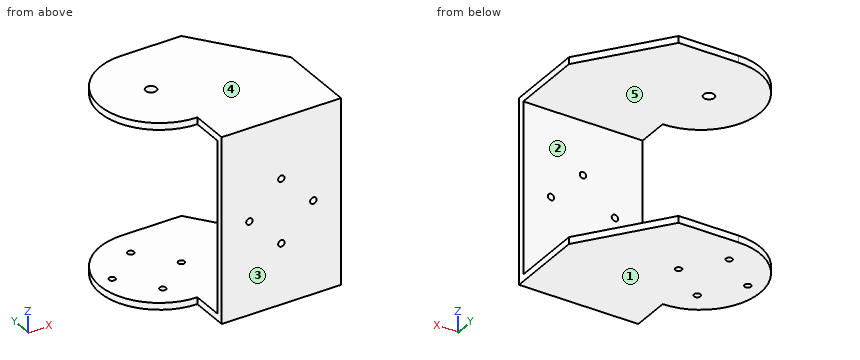
```python
from build123d import *

# Parameters (mm, degrees)
SKETCH1_W           = 28
SKETCH1_H           = 43.264
SKETCH1_R           = 0.75
BOSS_EXTRUDE1_DEPTH = 1.59
SKETCH2_W           = 28
SKETCH2_H           = 1.59
BOSS_EXTRUDE2_DEPTH = 35.41
BOSS_EXTRUDE5_DEPTH = 1.59
BOSS_EXTRUDE6_START = -1.59
BOSS_EXTRUDE6_DEPTH = 1.59
SKETCH9_R           = 0.75
CUT_EXTRUDE3_DEPTH  = 10
SKETCH10_R          = 1.25
CUT_EXTRUDE4_DEPTH  = 10
CUT_EXTRUDE5_REACH  = 65.441


with BuildPart() as part:
    # Sketch1 → Boss-Extrude1 (new body)
    with BuildSketch(Plane(origin=(0, 0, 0), x_dir=(1, 0, 0), z_dir=(0, 1, 0))):
        Rectangle(SKETCH1_W, SKETCH1_H)
        with Locations(Location((0, 7.5, 0), (0, 0, 90))):
            Circle(SKETCH1_R, mode=Mode.SUBTRACT)
        with Locations(Location((0, -7.5, 0), (0, 0, 90))):
            Circle(SKETCH1_R, mode=Mode.SUBTRACT)
        with Locations(Location((7.5, 0, 0), (0, 0, 90))):
            Circle(SKETCH1_R, mode=Mode.SUBTRACT)
        with Locations(Location((-7.5, 0, 0), (0, 0, 90))):
            Circle(SKETCH1_R, mode=Mode.SUBTRACT)
    extrude(amount=BOSS_EXTRUDE1_DEPTH)

    # Sketch2 → Boss-Extrude2 (add)
    with BuildSketch(Plane(origin=(0, 1.59, 0), x_dir=(1, 0, 0), z_dir=(0, 1, 0))):
        with Locations((0, 20.837)):
            Rectangle(SKETCH2_W, SKETCH2_H)
        with Locations((0, -20.837)):
            Rectangle(SKETCH2_W, SKETCH2_H)
    extrude(amount=BOSS_EXTRUDE2_DEPTH)

    # Sketch7 → Boss-Extrude5 (add)
    with BuildSketch(Plane(origin=(0, 0, -21.632), x_dir=(-1, 0, 0), z_dir=(0, 0, -1))):
        with BuildLine():
            Line((14, 37), (14, 9))
            ThreePointArc((14, 9), (28, 23), (14, 37))
        make_face()
    extrude(amount=-BOSS_EXTRUDE5_DEPTH)

    # Sketch8 → Boss-Extrude6 (add)
    with BuildSketch(Plane.XY.offset(21.632).offset(BOSS_EXTRUDE6_START)):
        with BuildLine():
            Line((-14, 37), (-14, 9))
            ThreePointArc((-14, 9), (-28, 23), (-14, 37))
        make_face()
    extrude(amount=BOSS_EXTRUDE6_DEPTH)

    # Sketch9 → Cut-Extrude3 (cut)
    with BuildSketch(Plane(origin=(0, 0, -21.632), x_dir=(-1, 0, 0), z_dir=(0, 0, -1))):
        with Locations((16, 30.5)):
            Circle(SKETCH9_R)
        with Locations((24.5, 24)):
            Circle(SKETCH9_R)
        with Locations((18, 15.5)):
            Circle(SKETCH9_R)
        with Locations((9.5, 22)):
            Circle(SKETCH9_R)
    extrude(amount=-CUT_EXTRUDE3_DEPTH, mode=Mode.SUBTRACT)

    # Sketch10 → Cut-Extrude4 (cut)
    with BuildSketch(Plane.XY.offset(21.632)):
        with Locations((-16, 23)):
            Circle(SKETCH10_R)
    extrude(amount=-CUT_EXTRUDE4_DEPTH, mode=Mode.SUBTRACT)

    # Cut-Extrude5: up to this face of the body (flat: up to its plane)
    cut_extrude5_end = Plane(part.part.faces().sort_by_distance((-4.502841696, 19.512586882, -21.632))[0])
    # Sketch11 → Cut-Extrude5 (cut, up to the picked face)
    with BuildSketch(Plane.XY.offset(21.632), mode=Mode.PRIVATE) as cut_extrude5_sk1:
        Polygon((0, 37), (14, 18.5), (14, 37), align=None)
    cut_extrude5_tool1 = split(extrude(cut_extrude5_sk1.sketch, amount=-CUT_EXTRUDE5_REACH, mode=Mode.PRIVATE), bisect_by=cut_extrude5_end, keep=Keep.BOTH, mode=Mode.PRIVATE)
    add(cut_extrude5_tool1.solids().sort_by(Axis((9.333333, 30.833333, 21.632), (0, 0, -1)))[0], mode=Mode.SUBTRACT)


solid = part.part
```
Work out the finished part from the listing and answer in its coordinate system (mm). Face numbers are marked on the shaded views. A direction names the side the tool comes from. Round coordinates to 2 decimals unless told otherwise and drop trailing zeros. Write each loop counter-clockwise with the first axis right and the second up, starting at its lowest first coordinate (ties: lowest second). Pieces come first, ordered by that corner, then holes.
1) Consider probe 1 along X at (y, z) = (1, 0); probe 2 along Z at (x, y) = (-15, 27); probe 3 along Y at (x, z) = (-13, 18). Determine where each line is inside the solid, lowest interval first.
2) Determine the mould class of the marked faces 3, 4 and 5 for opening direction Z: pulls with the +Z half, pulls with the -Z half, needs draft (parallel to the pull), parting line crosses it, or undercut.
3) A cutting plane is placed at D-D on x = -18. Determine the outline of the cut face in (y, z).
4) A cutting plane is placed at B-B on x = -7.5. Determine the outline of the cut face in (y, z), and give its area (3 significant figures).
5) Which of the six approach directions +Z, -Z, +X, -X, +Y, -Y give full straight-line access (tool end or side, diameter ignored) to the marked faces 1 and 2?
6) Flat-ended cylindrical pins translate along their axes: P1, Ø2.5, axis at y = 4.5, z = -5, coming from the -X side (3 decimals); P2, Ø2, axis at x = -11.5, z = -1.5, coming from the +Y side. Find the tip coordinate at first contact, or state that the pin passes through.
7) A cutting plane is placed at C-C on y = 32. Determine the outline of the cut face in (x, z).
8) A cutting plane is placed at A-A on z = 7.5. Determine the outline of the cut face in (x, y).
Entries:
1. probe 1: x = -14 to -8.25, -6.75 to 6.75, 8.25 to 14
1. probe 2: z = -21.63 to -20.04, 20.04 to 21.63
1. probe 3: y = 0 to 1.59
2. face 3: needs draft
2. face 4: pulls with the +Z half
2. face 5: undercut
3. outline: (9.58, -21.63) - (14.75, -21.63) - (14.75, -20.04) - (9.58, -20.04) - close; (9.58, 20.04) - (36.42, 20.04) - (36.42, 21.63) - (9.58, 21.63) - close; (16.25, -21.63) - (36.42, -21.63) - (36.42, -20.04) - (16.25, -20.04) - close
4. outline: (0, -21.63) - (37, -21.63) - (37, -20.04) - (1.59, -20.04) - (1.59, -0.75) - (0, -0.75) - close; (0, 0.75) - (1.59, 0.75) - (1.59, 20.04) - (37, 20.04) - (37, 21.63) - (0, 21.63) - close
4. area: 179 mm2
5. face 1: -Z, +X, -X, +Y, -Y
5. face 2: +X, -X, +Y
6. P1: passes through
6. P2: stops at y = 1.59
7. outline: (-24.72, -21.63) - (3.78, -21.63) - (3.78, -20.04) - (-24.72, -20.04) - close; (-24.72, 20.04) - (3.78, 20.04) - (3.78, 21.63) - (-24.72, 21.63) - close
8. outline: (-14, 0) - (-0.75, 0) - (-0.75, 1.59) - (-14, 1.59) - close; (0.75, 0) - (14, 0) - (14, 1.59) - (0.75, 1.59) - close
